from build123d import *

# Parameters (mm, degrees)
SKETCH1_R           = 25
BOSS_EXTRUDE1_DEPTH = 35
CUT_EXTRUDE1_DEPTH  = 34
SKETCH3_R           = 0.4
CUT_EXTRUDE2_DEPTH  = 78
SKETCH4_R           = 0.4
CUT_EXTRUDE3_DEPTH  = 22
SKETCH5_R           = 0.4
CUT_EXTRUDE4_DEPTH  = 10


with BuildPart() as part:
    # Sketch1 → Boss-Extrude1 (new body)
    with BuildSketch(Plane.XY):
        with BuildLine():
            Line((-30.39566951, 35), (30.39566951, 35))
            ThreePointArc((30.39566951, 35), (33.651422822, 33.651422822), (35, 30.39566951))
            Line((35, 30.39566951), (35, -30.39566951))
            ThreePointArc((35, -30.39566951), (33.651422822, -33.651422822), (30.39566951, -35))
            Line((30.39566951, -35), (-30.39566951, -35))
            ThreePointArc((-30.39566951, -35), (-33.651422822, -33.651422822), (-35, -30.39566951))
            Line((-35, -30.39566951), (-35, 30.39566951))
            ThreePointArc((-35, 30.39566951), (-33.651422822, 33.651422822), (-30.39566951, 35))
        make_face()
        Circle(SKETCH1_R, mode=Mode.SUBTRACT)
    extrude(amount=BOSS_EXTRUDE1_DEPTH)

    # Sketch2 → Cut-Extrude1 (cut)
    with BuildSketch(Plane.XY.offset(35)):
        with BuildLine():
            Line((-30.39566951, -34), (30.39566951, -34))
            ThreePointArc((30.39566951, -34), (32.944316041, -32.944316041), (34, -30.39566951))
            Line((34, -30.39566951), (34, 30.39566951))
            ThreePointArc((34, 30.39566951), (32.944316041, 32.944316041), (30.39566951, 34))
            Line((30.39566951, 34), (-30.39566951, 34))
            ThreePointArc((-30.39566951, 34), (-32.944316041, 32.944316041), (-34, 30.39566951))
            Line((-34, 30.39566951), (-34, -30.39566951))
            ThreePointArc((-34, -30.39566951), (-32.944316041, -32.944316041), (-30.39566951, -34))
        make_face()
    extrude(amount=-CUT_EXTRUDE1_DEPTH, mode=Mode.SUBTRACT)

    # Sketch3 → Cut-Extrude2 (cut)
    with BuildSketch(Plane(origin=(35, 0, 0), x_dir=(0, 0, -1), z_dir=(1, 0, 0))):
        with Locations(Location((-17.5, 20, 0), (0, 0, 90))):
            Circle(SKETCH3_R)
    extrude(amount=-CUT_EXTRUDE2_DEPTH, mode=Mode.SUBTRACT)

    # Sketch4 → Cut-Extrude3 (cut)
    with BuildSketch(Plane(origin=(0, 35, 0), x_dir=(1, 0, 0), z_dir=(0, 1, 0))):
        with Locations(Location((0, -17.5, 0), (0, 0, 270))):
            Circle(SKETCH4_R)
    extrude(amount=-CUT_EXTRUDE3_DEPTH, mode=Mode.SUBTRACT)

    # Sketch5 → Cut-Extrude4 (cut)
    with BuildSketch(Plane.XZ.offset(35)):
        with Locations(Location((-15, 17.5, 0), (0, 0, 270))):
            Circle(SKETCH5_R)
        with Locations(Location((15, 17.5, 0), (0, 0, 270))):
            Circle(SKETCH5_R)
    extrude(amount=-CUT_EXTRUDE4_DEPTH, mode=Mode.SUBTRACT)


solid = part.part
Geometry check sheet. Reference: the model listing, model coordinates, mm. A direction names the side the tool comes from. Round coordinates to 2 decimals unless told otherwise and drop trailing zeros. Loops run counter-clockwise (first coordinate to the right, second up) from the corner with the lowest first, then second, coordinate; pieces in that order, holes last. Notation, with made-up numbers: (72.5, 83) -> (124.5, 83) arc R21 ccw to (124.5, 103) -> close; hole circle Ø5 at (26.25, 7.25). An arc over 180 degrees is marked (long way). Answer as a JSON object with one key per item and string values. Group by question number.
Item 1: Thickness scan on line 1 along X through (y, z) = (0, 0.75); line 2 along Y through (x, z) = (-24.5, 32.5). Record the ranges inside material, lowest first.
Item 2: Cross-section at B-B, the plane y = 7. Record the cut outline in (x, z).
Item 3: Cross-section at D-D, the plane y = -28. Record the cut outline in (x, z), plus the area to 3 significant figures.
Item 4: Cross-section at C-C, the plane z = 33.5. Record the cut outline in (x, y), plus the area to 3 significant figures.
Item 5: Depth check by flat-ended pin: pin 1 Ø1 at (x, y) = (-23, 12) entering from +Z. Enter the tip coordinate at first touch or a pass-through.
Item 6: Cross-section at A-A, the plane x = 20. Record the cut outline in (y, z), plus the area to 3 significant figures.
Item 7: Set-up check for faces 5 (the face through (-32.92, 32.97, 18.24)), 6 (the face through (-33.7, 33.6, 17.3)): record each of +Z, -Z, +X, -X, +Y, -Y from which the full face is reachable in a straight line by a thin tool's end or side.
Item 8: Release check for a two-part mould opening along Y. For faces 1 (the face through (35, 0, 17)), 2 (the face through (-33.6, -33.7, 17.3)), 3 (the face through (0.4, 34, 18.2)), 4 (the face through (15, 23, 1)) record: pulls with the +Y half, pulls with the -Y half, needs draft (parallel to the pull), parting line crosses it, or undercut.
Determined:
{
 "1": {"line 1": "x = -35 to -25, 25 to 35", "line 2": "y = -35 to -34, 34 to 35"},
 "2": {"outline": "(-35, 0) -> (-24, 0) -> (-24, 1) -> (-34, 1) -> (-34, 35) -> (-35, 35) -> close; (24, 0) -> (35, 0) -> (35, 35) -> (34, 35) -> (34, 1) -> (24, 1) -> close"},
 "3": {"outline": "(-35, 0) -> (35, 0) -> (35, 35) -> (34, 35) -> (34, 1) -> (-34, 1) -> (-34, 35) -> (-35, 35) -> close", "area": "138 mm²"},
 "4": {"outline": "(-35, -30.4) arc R4.6 ccw to (-30.4, -35) -> (30.4, -35) arc R4.6 ccw to (35, -30.4) -> (35, 30.4) arc R4.6 ccw to (30.4, 35) -> (-30.4, 35) arc R4.6 ccw to (-35, 30.4) -> close; hole (-34, -30.4) arc R3.6 ccw to (-30.4, -34) -> (30.4, -34) arc R3.6 ccw to (34, -30.4) -> (34, 30.4) arc R3.6 ccw to (30.4, 34) -> (-30.4, 34) arc R3.6 ccw to (-34, 30.4) -> close", "area": "269 mm²"},
 "5": {"pin 1": "stops at z = 1"},
 "6": {"outline": "(-35, 0) -> (-15, 0) -> (-15, 1) -> (-34, 1) -> (-34, 35) -> (-35, 35) -> close; (15, 0) -> (35, 0) -> (35, 35) -> (34, 35) -> (34, 1) -> (15, 1) -> close", "area": "108 mm²"},
 "7": {"face 5": "+Z", "face 6": "+Z, -Z, -X, +Y"},
 "8": {"face 1": "needs draft", "face 2": "pulls with the -Y half", "face 3": "undercut", "face 4": "undercut"}
}
